For this review, take the finished solid that the model builds, in its own axes (mm). Face numbers are marked on the shaded views. A direction names the side the tool comes from. Coordinates: 2 decimals unless noted, no trailing zeros. Loops run counter-clockwise (first coordinate to the right, second up) from the corner with the lowest first, then second, coordinate; pieces in that order, holes last. Notation, with made-up numbers: M -7.75,74.25 L 0.25,74.25 A12 ccw 0.25,89.25 Z; hole C -32,5.25 d10. An arc over 180 degrees is marked long. Put each result on its own line as item: value.
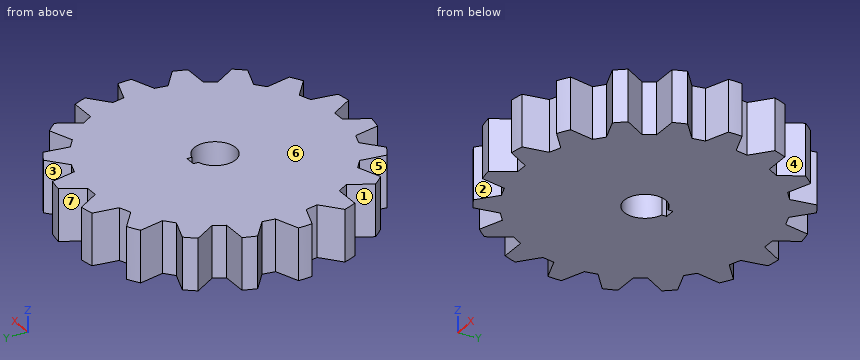
```python
from build123d import *

# Parameters (mm, degrees)
BOSS_EXTRUDE1_DEPTH = 25


with BuildPart() as part:
    # Sketch1 → Boss-Extrude1 (new body)
    with BuildSketch(Plane.XY):
        with BuildLine():
            Line((-3, 59.924953066), (3, 59.924953066))
            Line((3, 59.924953066), (9.05913636, 70.419685092))
            ThreePointArc((9.05913636, 70.419685092), (12.329020614, 69.921350464), (15.5721472, 69.271265555))
            Line((15.5721472, 69.271265555), (17.676463174, 57.337096627))
            Line((17.676463174, 57.337096627), (23.314618899, 55.284975767))
            Line((23.314618899, 55.284975767), (32.597754376, 63.074451322))
            ThreePointArc((32.597754376, 63.074451322), (35.5, 61.487803669), (38.325199987, 59.767709057))
            Line((38.325199987, 59.767709057), (36.220884013, 47.83354013))
            Line((36.220884013, 47.83354013), (40.817150671, 43.976814472))
            Line((40.817150671, 43.976814472), (52.204602123, 48.121507844))
            ThreePointArc((52.204602123, 48.121507844), (54.389155461, 45.637920288), (56.455668036, 43.05528477))
            Line((56.455668036, 43.05528477), (50.396531676, 32.560552745))
            Line((50.396531676, 32.560552745), (53.396531676, 27.364400322))
            Line((53.396531676, 27.364400322), (65.514804396, 27.364400322))
            ThreePointArc((65.514804396, 27.364400322), (66.718176076, 24.283430176), (67.776749323, 21.149757711))
            Line((67.776749323, 21.149757711), (58.493613846, 13.360282156))
            Line((58.493613846, 13.360282156), (59.535502912, 7.451435638))
            Line((59.535502912, 7.451435638), (70.922954363, 3.306742265))
            ThreePointArc((70.922954363, 3.306742265), (71, 0), (70.922954363, -3.306742265))
            Line((70.922954363, -3.306742265), (59.535502912, -7.451435638))
            Line((59.535502912, -7.451435638), (58.493613846, -13.360282156))
            Line((58.493613846, -13.360282156), (67.776749323, -21.149757711))
            ThreePointArc((67.776749323, -21.149757711), (66.718176076, -24.283430176), (65.514804396, -27.364400322))
            Line((65.514804396, -27.364400322), (53.396531676, -27.364400322))
            Line((53.396531676, -27.364400322), (50.396531676, -32.560552745))
            Line((50.396531676, -32.560552745), (56.455668036, -43.05528477))
            ThreePointArc((56.455668036, -43.05528477), (54.389155461, -45.637920288), (52.204602123, -48.121507844))
            Line((52.204602123, -48.121507844), (40.817150671, -43.976814472))
            Line((40.817150671, -43.976814472), (36.220884013, -47.83354013))
            Line((36.220884013, -47.83354013), (38.325199987, -59.767709057))
            ThreePointArc((38.325199987, -59.767709057), (35.5, -61.487803669), (32.597754376, -63.074451322))
            Line((32.597754376, -63.074451322), (23.314618899, -55.284975767))
            Line((23.314618899, -55.284975767), (17.676463174, -57.337096627))
            Line((17.676463174, -57.337096627), (15.5721472, -69.271265555))
            ThreePointArc((15.5721472, -69.271265555), (12.329020614, -69.921350464), (9.05913636, -70.419685092))
            Line((9.05913636, -70.419685092), (3, -59.924953066))
            Line((3, -59.924953066), (-3, -59.924953066))
            Line((-3, -59.924953066), (-9.05913636, -70.419685092))
            ThreePointArc((-9.05913636, -70.419685092), (-12.329020614, -69.921350464), (-15.5721472, -69.271265555))
            Line((-15.5721472, -69.271265555), (-17.676463174, -57.337096627))
            Line((-17.676463174, -57.337096627), (-23.314618899, -55.284975767))
            Line((-23.314618899, -55.284975767), (-32.597754376, -63.074451322))
            ThreePointArc((-32.597754376, -63.074451322), (-35.5, -61.487803669), (-38.325199987, -59.767709057))
            Line((-38.325199987, -59.767709057), (-36.220884013, -47.83354013))
            Line((-36.220884013, -47.83354013), (-40.817150671, -43.976814472))
            Line((-40.817150671, -43.976814472), (-52.204602123, -48.121507844))
            ThreePointArc((-52.204602123, -48.121507844), (-54.389155461, -45.637920288), (-56.455668036, -43.05528477))
            Line((-56.455668036, -43.05528477), (-50.396531676, -32.560552745))
            Line((-50.396531676, -32.560552745), (-53.396531676, -27.364400322))
            Line((-53.396531676, -27.364400322), (-65.514804396, -27.364400322))
            ThreePointArc((-65.514804396, -27.364400322), (-66.718176076, -24.283430176), (-67.776749323, -21.149757711))
            Line((-67.776749323, -21.149757711), (-58.493613846, -13.360282156))
            Line((-58.493613846, -13.360282156), (-59.535502912, -7.451435638))
            Line((-59.535502912, -7.451435638), (-70.922954363, -3.306742265))
            ThreePointArc((-70.922954363, -3.306742265), (-71, 0), (-70.922954363, 3.306742265))
            Line((-70.922954363, 3.306742265), (-59.535502912, 7.451435638))
            Line((-59.535502912, 7.451435638), (-58.493613846, 13.360282156))
            Line((-58.493613846, 13.360282156), (-67.776749323, 21.149757711))
            ThreePointArc((-67.776749323, 21.149757711), (-66.718176076, 24.283430176), (-65.514804396, 27.364400322))
            Line((-65.514804396, 27.364400322), (-53.396531676, 27.364400322))
            Line((-53.396531676, 27.364400322), (-50.396531676, 32.560552745))
            Line((-50.396531676, 32.560552745), (-56.455668036, 43.05528477))
            ThreePointArc((-56.455668036, 43.05528477), (-54.389155461, 45.637920288), (-52.204602123, 48.121507844))
            Line((-52.204602123, 48.121507844), (-40.817150671, 43.976814472))
            Line((-40.817150671, 43.976814472), (-36.220884013, 47.83354013))
            Line((-36.220884013, 47.83354013), (-38.325199987, 59.767709057))
            ThreePointArc((-38.325199987, 59.767709057), (-35.5, 61.487803669), (-32.597754376, 63.074451322))
            Line((-32.597754376, 63.074451322), (-23.314618899, 55.284975767))
            Line((-23.314618899, 55.284975767), (-17.676463174, 57.337096627))
            Line((-17.676463174, 57.337096627), (-15.5721472, 69.271265555))
            ThreePointArc((-15.5721472, 69.271265555), (-12.329020614, 69.921350464), (-9.05913636, 70.419685092))
            Line((-9.05913636, 70.419685092), (-3, 59.924953066))
        make_face()
        with BuildLine():
            Line((2.5, 9.682458366), (2.5, 12))
            Line((2.5, 12), (-2.5, 12))
            Line((-2.5, 12), (-2.5, 9.682458366))
            ThreePointArc((-2.5, 9.682458366), (0, -10), (2.5, 9.682458366))
        make_face(mode=Mode.SUBTRACT)
    extrude(amount=-BOSS_EXTRUDE1_DEPTH)


solid = part.part
```
(1) Add section A-A (y = 0). Write out the cut boundary in (x, z).
Determined:
outline: M -71,-25 L -10,-25 L -10,0 L -71,0 Z; M 10,-25 L 71,-25 L 71,0 L 10,0 Z
(2) Tool access review of the marked faces 1, 2, 3 and 4: name each direction out of +Z, -Z, +X, -X, +Y, -Y from which nothing blocks a thin tool from reaching the whole face with its end or side.
Determined:
face 1: +Z, -Z, -X
face 2: +Z, -Z, -Y
face 3: +Z, -Z, +Y
face 4: +Z, -Z, +X
(3) Draft analysis for pull direction Y (two halves, no side actions). For the marked faces 5, 6 and 7, state which applies: +Y half, -Y half, draft (parallel to the pull), parting line (faces both ways), or undercut.
Determined:
face 5: undercut
face 6: draft
face 7: +Y half
(4) Add section B-B (x = 0). Write out the cut boundary in (y, z).
Determined:
outline: M -59.92,-25 L -10,-25 L -10,0 L -59.92,0 Z; M 12,-25 L 59.92,-25 L 59.92,0 L 12,0 Z
(5) For pin 1 (10 mm diameter, centred on y = -2, z = -18, fed in from -X); pin 2 (9.5 mm diameter, centred on x = -56.5, z = -7.5, fed in from +Y); pin 3 (13.5 mm diameter, centred on x = 58, z = -6.5, fed in from -Y); pin 4 (3.5 mm diameter, centred on x = -59.5, z = -18.5, fed in from -Y), all flat-tipped, find the tip position at first contact; note any pin that passes through.
Determined:
pin 1: stops at x = -71
pin 2: stops at y = 48.12
pin 3: stops at y = -48.12
pin 4: stops at y = -27.36
(6) Wall thickness on line 1 along Y through (x, z) = (0, -5.25); line 2 along Y through (x, z) = (55, -16.75); line 3 along X through (y, z) = (0.5, -23): over which ranges is each line inside the solid? List them lowest first. Write a range as [from, to].
Determined:
line 1: y = [-59.92, -10], [12, 59.92]
line 2: y = [-44.9, -40.53], [-27.36, 27.36], [40.53, 44.9]
line 3: x = [-71, -9.99], [9.99, 71]
